Geometry check sheet. Reference: the model listing, model coordinates, mm. A direction names the side the tool comes from. Give positions to 0.01 mm unless a question says otherwise; leave off trailing zeros. Write each loop counter-clockwise with the first axis right and the second up, starting at its lowest first coordinate (ties: lowest second). Pieces come first, ordered by that corner, then holes. Notation, with made-up numbers: (39, 15) - (65, 15) arc R14 ccw to (65, 23) - close; hole circle Ø1 at (17, -34.75). An arc over 180 degrees is marked (long way). Write item = value, one per line. Start each with the question number.
(1) Depth check by flat-ended pin: pin 1 Ø8 at (y, z) = (24.5, 21.5) entering from -X; pin 2 Ø5 at (x, z) = (59, 44) entering from -Y; pin 3 Ø1.5 at (x, z) = (48.5, 19.5) entering from +Y; pin 4 Ø13 at (y, z) = (32, 25) entering from +X. Enter the tip coordinate at first touch or a pass-through.
(2) Section check C-C, the plane x = 59. Enter the section's corners in (y, z), plus the area to 3 significant figures.
(3) Section check D-D, the plane z = 17.5. Enter the section's corners in (x, y), plus the area to 3 significant figures.
(4) Thickness scan on L1, parallel to X at y = -2, z = 44; L2, parallel to Z at x = 8, y = -2.75; L3, parallel to Y at x = 24.5, z = 25. Record the ranges inside material, lowest first.
(5) Section check A-A, the plane y = 5. Enter the section's corners in (x, z), plus the area to 3 significant figures.
(6) Draft check along Y on faces 1 (the cylindrical face through (23, 32, 20)), 2 (the flat face through (56, 0, 26)), 3 (the flat face through (0, -2, 26)), 4 (the cylindrical face through (43, 32, 20)). Enter one of: pulls with the +Y half, pulls with the -Y half, needs draft (parallel to the pull), parting line crosses it, or undercut.
(7) Access from +Z, -Z, +X, -X, +Y, -Y to the whole of each face (thin tool, end or side, straight path). Record for faces 5 (the flat face through (21.5, 20, 26)), 6 (the flat face through (67, -2, 26)), 7 (the flat face through (23, 40, 26)), 8 (the flat face through (25.5, 20, 26)), 9 (the flat face through (45.5, 20, 26)).
(8) Section check B-B, the plane z = 25. Enter the section's corners in (x, y), plus the area to 3 significant figures.
Autodesk Inventor part; units mm, degrees
ref_plane "YZ Plane" through (0, 0, 0) normal (1, 0, 0) x (0, 1, 0)
ref_plane "XZ Plane" through (0, 0, 0) normal (0, 1, 0) x (-1, 0, 0)
ref_plane "XY Plane" through (0, 0, 0) normal (0, 0, 1) x (1, 0, 0)
sketch "Sketch1" plane through (0, 0, 0) normal (0, 0, 1) x (1, 0, 0)
  line L0 (0, 0) -> (67, 0)
  line L1 (67, 0) -> (67, -4)
  line L2 (67, -4) -> (0, -4)
  line L3 (0, -4) -> (0, 0)
  dimension "d0" = 67
  dimension "d1" = 4
extrude "Extrusion1" add sketch "Sketch1" along normal blind 52
sketch "Sketch2" plane through (0, 0, 0) normal (0, 1, 0) x (1, 0, 0)
  line L0 (8, -44) -> (59, -44)
  line L1 (59, -44) -> (59, -8)
  line L2 (59, -8) -> (8, -8)
  line L3 (8, -8) -> (8, -44)
  line L4 (8, -44) -> (59, -8) construction
  line L5 (59, -44) -> (8, -8) construction
  line L6 (0, 0) -> (0, -52)
  line L7 (0, 0) -> (67, 0)
  circle A0 centre (8, -8) radius 3.25
  circle A1 centre (59, -8) radius 3.25
  circle A2 centre (8, -44) radius 3.25
  circle A3 centre (59, -44) radius 3.25
  point P0 (33.5, -26)
  dimension "d4" = 51
  dimension "d5" = 36
  dimension "d6" = 8
  dimension "d7" = 8
  dimension "d8" = 6.5
  dimension "d9" = 6.5
  dimension "d10" = 6.5
  dimension "d11" = 6.5
extrude "Extrusion2" cut sketch "Sketch2" against normal blind 4 contours L3 A2 L0 | L0 A2 L3 | A3 L1 L0 | L0 L1 A3 | A0 L2 L3 | L3 L2 A0 | A1 L2 L1 | L1 L2 A1
sketch "Sketch3" plane through (0, 0, 0) normal (0, 1, 0) x (1, 0, 0)
  line L0 (0, -52) -> (67, -52)
  line L1 (21.5, 0) -> (25.5, 0)
  line L2 (25.5, 0) -> (25.5, -52)
  line L3 (25.5, -52) -> (21.5, -52)
  line L4 (21.5, -52) -> (21.5, 0)
  line L5 (0, 0) -> (0, -52)
  line L6 (45.5, 0) -> (41.5, 0)
  line L7 (41.5, 0) -> (41.5, -52)
  line L8 (41.5, -52) -> (45.5, -52)
  line L9 (45.5, -52) -> (45.5, 0)
  line L10 (67, 0) -> (67, -52)
  dimension "d14" = 4
  dimension "d15" = 21.5
  dimension "d16" = 4
  dimension "d17" = 21.5
  dimension "d18" = 52
  dimension "d19" = 52
extrude "Extrusion3" add sketch "Sketch3" along normal blind 40
sketch "Sketch4" plane through (21.5, 0, 0) normal (-1, 0, 0) x (0, 0, 1)
  circle A0 centre (25, 32) radius 5
  line L0 (0, -4) -> (52, -4)
  line L1 (52, 0) -> (52, 40)
  point P0 (0, 0)
  dimension "d22" = 10
  dimension "d23" = 36
  dimension "d24" = 27
extrude "Extrusion4" cut sketch "Sketch4" against normal blind 40
properties part number "SDB 32" material "Stainless Steel"
Model answer:
q1.pin_1 = 21.5
q1.pin_2 = through
q1.pin_3 = 0
q1.pin_4 = 45.5
q2.outline = (-4, 0) - (0, 0) - (0, 4.75) - (-4, 4.75) - close; (-4, 11.25) - (0, 11.25) - (0, 40.75) - (-4, 40.75) - close; (-4, 47.25) - (0, 47.25) - (0, 52) - (-4, 52) - close
q2.area = 156 mm²
q3.outline = (0, -4) - (67, -4) - (67, 0) - (45.5, 0) - (45.5, 40) - (41.5, 40) - (41.5, 0) - (25.5, 0) - (25.5, 40) - (21.5, 40) - (21.5, 0) - (0, 0) - close
q3.area = 588 mm²
q4.L1 = 0 to 4.75, 11.25 to 55.75, 62.25 to 67
q4.L2 = 0 to 4.75, 11.25 to 40.75, 47.25 to 52
q4.L3 = -4 to 27, 37 to 40
q5.outline = (21.5, 0) - (25.5, 0) - (25.5, 52) - (21.5, 52) - close; (41.5, 0) - (45.5, 0) - (45.5, 52) - (41.5, 52) - close
q5.area = 416 mm²
q6.face_1 = undercut
q6.face_2 = pulls with the +Y half
q6.face_3 = needs draft
q6.face_4 = undercut
q7.face_5 = +Z, -Z, -X, +Y
q7.face_6 = +Z, -Z, +X, +Y, -Y
q7.face_7 = +Z, -Z, +X, -X, +Y
q7.face_8 = +Z, -Z, +Y
q7.face_9 = +Z, -Z, +X, +Y
q8.outline = (0, -4) - (67, -4) - (67, 0) - (45.5, 0) - (45.5, 27) - (41.5, 27) - (41.5, 0) - (25.5, 0) - (25.5, 27) - (21.5, 27) - (21.5, 0) - (0, 0) - close; (21.5, 37) - (25.5, 37) - (25.5, 40) - (21.5, 40) - close; (41.5, 37) - (45.5, 37) - (45.5, 40) - (41.5, 40) - close
q8.area = 508 mm²
